Verification items for the finished model (mm, model axes). Face numbers are marked on the shaded views. A direction names the side the tool comes from. Coordinates: 2 decimals unless noted, no trailing zeros. Write each loop counter-clockwise with the first axis right and the second up, starting at its lowest first coordinate (ties: lowest second). Pieces come first, ordered by that corner, then holes. Notation, with made-up numbers: (-14.75, -8) - (19.25, -8) arc R31 ccw to (19.25, 27) - close; hole circle Ø4 at (47.5, 14.5). An arc over 180 degrees is marked (long way). Use CSV: the item, a comma, the result in double quotes. Start each with the question number.
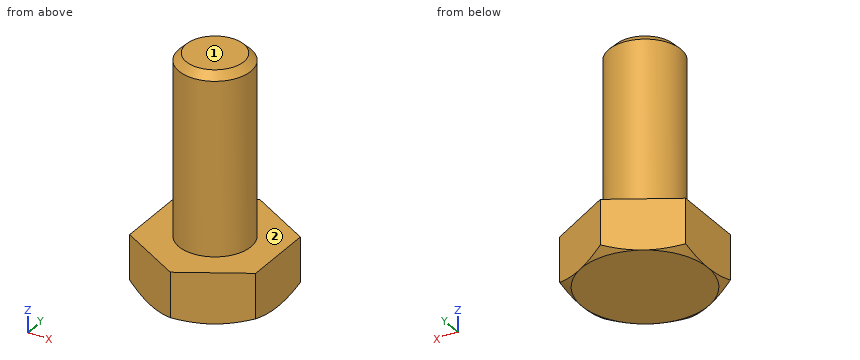
```python
from build123d import *

# Parameters (mm, degrees)
ESQUISSE1_W        = 2
ESQUISSE1_H        = 10
BOSS_EXTRU_1_DEPTH = 2.8


with BuildPart() as part:
    # Esquisse1 → Base-Révolution (revolve)
    with BuildSketch(Plane(origin=(0, 0, 0), x_dir=(1, 0, 0), z_dir=(0, 1, 0))):
        with Locations((1, -5)):
            Rectangle(ESQUISSE1_W, ESQUISSE1_H)
    revolve(axis=Axis((0, 0, 0), (0, 0, 1)))

    # Chanfrein1: read off the stored shape, not the designer's step
    # Chanfrein1 outline → Chanfrein1 (revolve, cut)
    with BuildSketch(Plane.XZ):
        Polygon((2, 10), (1.6, 10), (2, 9.6), align=None)
    revolve(axis=Axis((0, 0, 0), (0, 0, 1)), mode=Mode.SUBTRACT)

    # Esquisse6 → Boss.-Extru.1 (add)
    with BuildSketch(Plane.XY):
        Polygon((3.5, -2.020725942), (3.5, 2.020725942), (0, 4.041451884), (-3.5, 2.020725942), (-3.5, -2.020725942), (0, -4.041451884), align=None)
    extrude(amount=-BOSS_EXTRU_1_DEPTH)

    # Esquisse7 → Enlèvement de matière-Révolution1 (revolve, cut)
    with BuildSketch(Plane(origin=(0, 0, 0), x_dir=(1, 0, 0), z_dir=(0, 1, 0))):
        Polygon((-3.5, 2.8), (-8.349742261, 2.8), (-8.349742261, 0), align=None)
    revolve(axis=Axis((0, 0, -6.239446496), (0, 0, 1)), mode=Mode.SUBTRACT)


solid = part.part
```
Q1. Scan lines: line 1 along Z through (x, y) = (-1.25, -2.5); line 2 along X through (y, z) = (0.5, 3.5); line 3 along Y through (x, z) = (-1.25, 4). Record each from-to range of solid material in increasing order. Write a range as from..to.
Q2. Gauge pin test, flat ends, axial feed: pin 1 (1 mm diameter, centred on y = 2, z = 6.5, fed in from +X); pin 2 (2 mm diameter, centred on x = -2, z = 2, fed in from -Y); pin 3 (4 mm diameter, centred on y = 2.5, z = 8, fed in from -X). Record the tip position at first contact, or that the pin passes through.
Q3. Cross-section at A-A (z = 2.75). Record the cut outline in (x, y).
Q4. Tool access check on the marked faces 1 and 2. Record the directions out of +Z, -Z, +X, -X, +Y, -Y that give a thin tool (end or side, any length) a straight path to the whole face; none if there is none.
Reply:
1,line 1,"-2.8..0"
1,line 2,"-1.94..1.94"
1,line 3,"-1.56..1.56"
2,pin 1,"x = 1.32"
2,pin 2,"y = -1.73"
2,pin 3,"x = -1.94"
3,outline,"circle Ø4 at (0, 0)"
4,face 1,"+Z, +X, -X, +Y, -Y"
4,face 2,"+Z"
